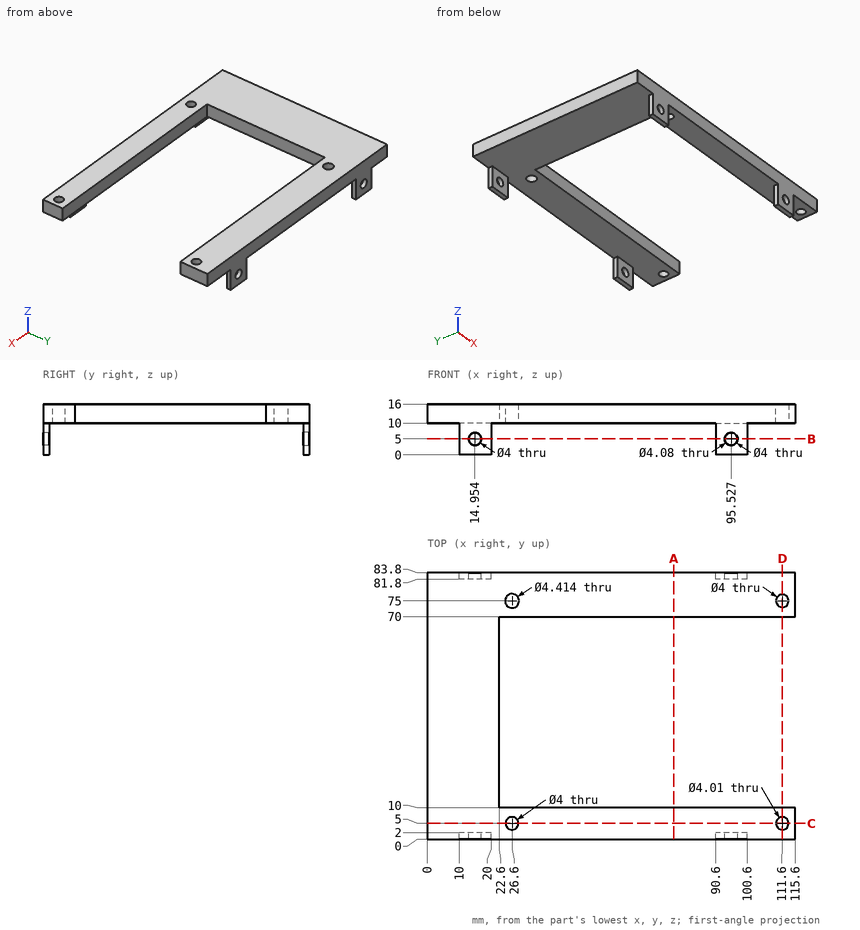
The drawing under review shows one solid part. Ordinate dimensions are in mm from its lowest x, y, z. Give positions to 0.01 mm unless a question says otherwise; leave off trailing zeros. Write each loop counter-clockwise with the first axis right and the second up, starting at its lowest first coordinate (ties: lowest second). Pieces come first, ordered by that corner, then holes. Notation, with made-up numbers: M 68.25,37 L 115.25,37 A25 cw 115.25,67 Z; hole C -36.75,22.25 d5. An arc over 180 degrees is marked long. Write each question's results on one line, items separated by ' | '. Start each with the question number.
1. We need section A-A (x = 77.5). Write out the cut boundary in (y, z).
2. We need section C-C (y = 5). Write out the cut boundary in (x, z) (1 decimal).
3. We need section D-D (x = 111.6). Write out the cut boundary in (y, z) (1 decimal).
4. We need section B-B (z = 5). Count the separate pieces of the cut face and the enclosed holes in it.
5. For probe 1 along Y at (x, z) = (26.6, 11.3); probe 2 along Y at (x, z) = (105, 12.75); probe 3 along X at (y, z) = (1.35, 5), list the stretches that pass through material, from the lowest coordinate up. Write a range as [from, to].
6. Insertion check: pin 1 Ø4 at (y, z) = (17, 7.5) entering from +X; pin 2 Ø1 at (y, z) = (0.5, 6.5) entering from +X; pin 3 Ø6.5 at (y, z) = (52.5, 13.5) entering from +X; pin 4 Ø2 at (y, z) = (1.5, 7.5) entering from -X. Each pin has a flat end and moves straight along its axis. Give the tip position at first contact, or say it passes through.
Results found:
1) outline: M 0,10 L 10,10 L 10,16 L 0,16 Z; M 70,10 L 83.8,10 L 83.8,16 L 70,16 Z
2) outline: M 0,10 L 24.6,10 L 24.6,16 L 0,16 Z; M 28.6,10 L 109.6,10 L 109.6,16 L 28.6,16 Z; M 113.6,10 L 115.6,10 L 115.6,16 L 113.6,16 Z
3) outline: M 0,10 L 3,10 L 3,16 L 0,16 Z; M 7,10 L 10,10 L 10,16 L 7,16 Z; M 70,10 L 73,10 L 73,16 L 70,16 Z; M 77,10 L 83.8,10 L 83.8,16 L 77,16 Z
4) separate pieces: 8 | enclosed holes: 0
5) probe 1: y = [0, 3], [7, 10], [70, 72.79], [77.21, 83.8] | probe 2: y = [0, 10], [70, 83.8] | probe 3: x = [10, 12.95], [16.95, 20], [90.6, 93.53], [97.53, 100.6]
6) pin 1: passes through | pin 2: stops at x = 100.6 | pin 3: stops at x = 22.6 | pin 4: stops at x = 10
